from build123d import *

# Parameters (mm, degrees)
PAD_DEPTH           = 100
SKETCH001_W         = 40
SKETCH001_H         = 3
POCKET_DEPTH        = 60
LINEARPATTERN_COUNT = 18
LINEARPATTERN_PITCH = 5.705882
FILLET_R            = 1


with BuildPart() as part:
    # Sketch → Pad (new body)
    with BuildSketch(Plane.XY):
        Polygon((-3, 0), (-3, 50), (0, 50), (0, 0), (0, -50), align=None)
    extrude(amount=PAD_DEPTH)

    # Sketch001 → Pocket (cut)
    with BuildSketch(Plane.XZ):
        with Locations((-0.275086, 4.5)):
            Rectangle(SKETCH001_W, SKETCH001_H)
    pocket = extrude(amount=POCKET_DEPTH, mode=Mode.SUBTRACT)

    # LinearPattern: Pocket ×18
    with Locations(*[(0, 0, i * LINEARPATTERN_PITCH) for i in range(1, LINEARPATTERN_COUNT)]):
        add(pocket, mode=Mode.SUBTRACT)

    # Fillet
    fillet_edges = [part.edges().sort_by_distance(p)[0] for p in [
        (-3, 50, 50),
        (0, 50, 50),
        (-1.5, 50, 0),
        (-1.5, 50, 100),
    ]]
    fillet(fillet_edges, radius=FILLET_R)


solid = part.part
Design review of the part built by this model. Coordinates are the model's own, in mm. A direction names the side the tool comes from. Coordinates: 2 decimals unless noted, no trailing zeros. Use a Markdown table: item, result. Add a question column.
Item 1: Wall thickness on L1, parallel to X at y = -33, z = 76.5; L2, parallel to Y at x = -1.8, z = 84; L3, parallel to X at y = -15, z = 82: over which ranges is each line inside the solid? List them lowest first. Write a range as from..to.
Item 2: Clearance check with a flat-ended pin moving along its axis: P1, Ø0.9, axis at x = -2, z = 16, coming from the -Y side. State where the tip first meets the part, or that it passes through.
Item 3: We need section A-A, the plane y = -25.5. Count the separate pieces of the cut face and the enclosed holes in it, and give its area (3 significant figures).
Item 4: The part is to be moulded in two halves that separate along Z. For faces 1 (the flat face through (0, 21, 60)), 2 (the flat face through (-1, -14, 45.941)), say which applies: +Z half, -Z half, draft (parallel to the pull), parting line (faces both ways), or undercut.
Item 5: Machinability: for faces 3 (the flat face through (-2, 0, 16)), 4 (the flat face through (-1.48, -25.35, 41.57)), which of the approach directions +Z, -Z, +X, -X, +Y, -Y give a long, thin tool a straight path to every point of the face, cutting with its end or side? Answer none if there is none.
Numbers:
| question | item | result |
|---|---|---|
| 1 | L1 | x = -1.02..0 |
| 1 | L2 | y = 0..50 |
| 1 | L3 | x = -2.1..0 |
| 2 | P1 | stops at y = 0 |
| 3 | separate pieces | 18 |
| 3 | enclosed holes | 0 |
| 3 | area | 72.0 mm^2 |
| 4 | face 1 | draft |
| 4 | face 2 | undercut |
| 5 | face 3 | +X, -X, -Y |
| 5 | face 4 | +Z, -Z, -X, -Y |
